Geometry: see drawing. Coordinates: mm, zero at the bounding-box minimum. A direction names the side the tool comes from. Give positions to 0.01 mm unless a question says otherwise; leave off trailing zeros. Write each loop counter-clockwise with the first axis right and the second up, starting at its lowest first coordinate (ties: lowest second). Pieces come first, ordered by that corner, then holes. Notation, with made-up numbers: (19.5, 7) - (77.5, 7) arc R10 cw to (77.5, 23) - close; hole circle Ø3 at (55.5, 71). An arc over 180 degrees is marked (long way). Return JSON: item names as keys, results as strings.
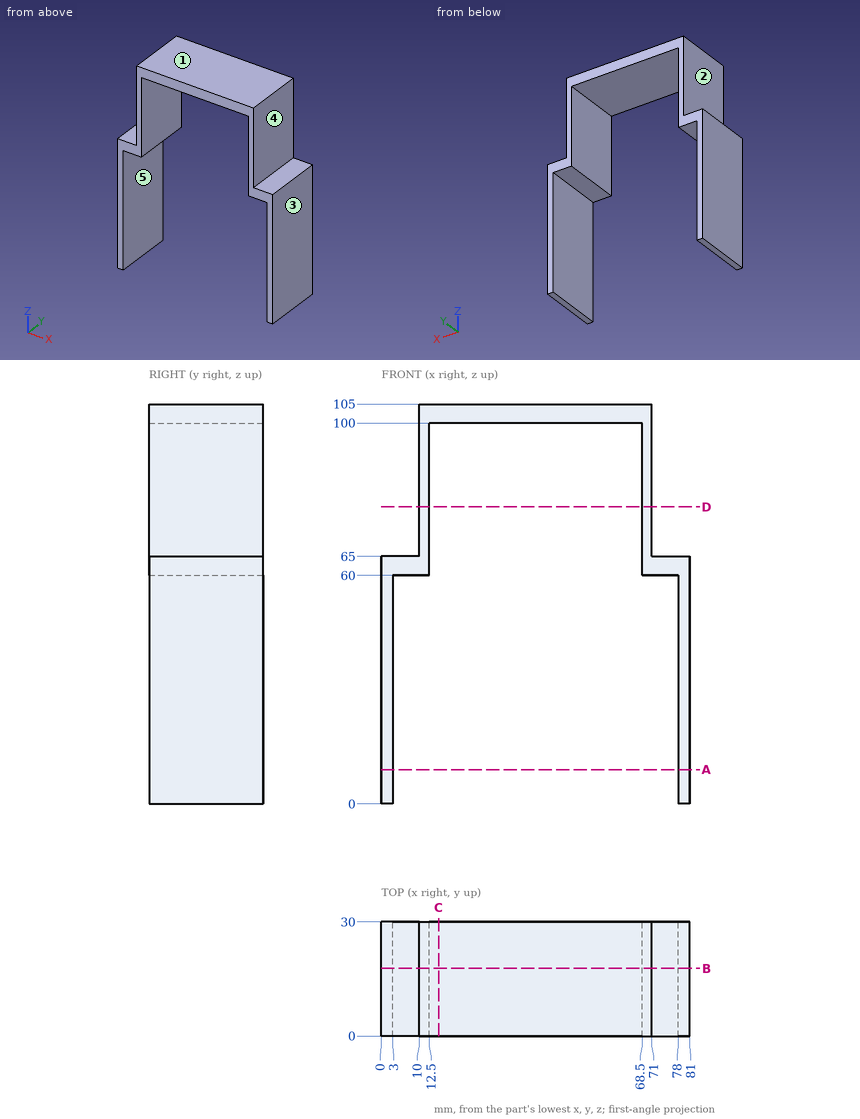
Q1. Section query C-C, the plane x = 15. Return the cut outline in (y, z).
Answer key:
{"outline": "(0, 100) - (30, 100) - (30, 105) - (0, 105) - close"}
Q2. Pin query (flat end, axial travel): P1, Ø9, axis at y = 20.5, z = 78, coming from the -X side; P2, Ø7.5, axis at x = 9.5, y = 10.5, coming from the -Z side; P3, Ø12, axis at x = 38, y = 25.5, coming from the -Z side; P4, Ø8, axis at x = 74.5, y = 14.5, coming from the +Z side. Return the tip coordinate at first contact, or that it passes through.
Answer key:
{"P1": "stops at x = 10", "P2": "stops at z = 60", "P3": "stops at z = 100", "P4": "stops at z = 105"}
Q3. Set-up query: the marked faces 1, 2, 3, 4 and 5. Return all of +Z, -Z, +X, -X, +Y, -Y with unobstructed straight access to the full face (end or side cutting, diameter ignored); none if empty.
Answer key:
{"face 1": "+Z, +X, -X, +Y, -Y", "face 2": "+Z, -X, +Y, -Y", "face 3": "+Z, -Z, +X, +Y, -Y", "face 4": "+Z, +X, +Y, -Y", "face 5": "-Z, +Y, -Y"}
Q4. Section query D-D, the plane z = 78. Return the cut outline in (x, y), plus the area to 3 significant figures.
Answer key:
{"outline": "(10, 0) - (12.5, 0) - (12.5, 30) - (10, 30) - close; (68.5, 0) - (71, 0) - (71, 30) - (68.5, 30) - close", "area": "150 mm^2"}
Q5. Section query B-B, the plane y = 17.75. Return the cut outline in (x, z), plus the area to 3 significant figures.
Answer key:
{"outline": "(0, 0) - (3, 0) - (3, 60) - (12.5, 60) - (12.5, 100) - (68.5, 100) - (68.5, 60) - (78, 60) - (78, 0) - (81, 0) - (81, 65) - (71, 65) - (71, 105) - (10, 105) - (10, 65) - (0, 65) - close", "area": "965 mm^2"}
Q6. Material intervals for probe 1 along X at (y, z) = (8, 51); probe 2 along X at (y, z) = (11, 97); probe 3 along Z at (x, y) = (71.5, 20.75), sorted ascending. Write a range as [from, to].
Answer key:
{"probe 1": "x = [0, 3], [78, 81]", "probe 2": "x = [10, 12.5], [68.5, 71]", "probe 3": "z = [60, 65]"}
Q7. Section query A-A, the plane z = 9. Return the cut outline in (x, y).
Answer key:
{"outline": "(0, 0) - (3, 0) - (3, 30) - (0, 30) - close; (78, 0) - (81, 0) - (81, 30) - (78, 30) - close"}
